The model under review builds one solid part; all positions refer to its coordinate system, in mm. A direction names the side the tool comes from. Coordinates: 2 decimals unless noted, no trailing zeros. Write each loop counter-clockwise with the first axis right and the second up, starting at its lowest first coordinate (ties: lowest second). Pieces come first, ordered by that corner, then holes. Notation, with made-up numbers: (-36.5, -2.75) - (-25.5, -2.75) arc R31 ccw to (-25.5, 34.25) - close; hole circle Ø9 at (-10, 41). An arc over 180 degrees is marked (long way). Answer as CSV lines item,"result". Start each with the question number.
```python
from build123d import *

# Parameters (mm, degrees)
SKETCH_1_R          = 2.5
EXTRUDE_1_DEPTH     = 1.5
SKETCH_3_R          = 6
EXTRUDE_2_DEPTH     = 1.5
SKETCH_4_R          = 4.5
EXTRUDE_3_DEPTH     = 6
SKETCH_5_R          = 3.25
EXTRUDE_4_DEPTH     = 1
CHAMFER_1_SIZE      = 0.5
CUT_EXTRUDE_1_REACH = 15.115
SKETCH_6_W          = 35.44
SKETCH_6_H          = 3.5


with BuildPart() as part:
    # 草图1 → 凸台-拉伸1 (new body)
    with BuildSketch(Plane.XY):
        Circle(SKETCH_1_R)
    extrude(amount=EXTRUDE_1_DEPTH)

    # 草图3 → 凸台-拉伸2 (add)
    with BuildSketch(Plane.XY.offset(1.5)):
        Circle(SKETCH_3_R)
    extrude(amount=EXTRUDE_2_DEPTH)

    # 草图4 → 凸台-拉伸3 (add)
    with BuildSketch(Plane.XY.offset(3)):
        Circle(SKETCH_4_R)
    extrude(amount=EXTRUDE_3_DEPTH)

    # 草图5 → 凸台-拉伸4 (add)
    with BuildSketch(Plane.XY.offset(9)):
        Circle(SKETCH_5_R)
    extrude(amount=EXTRUDE_4_DEPTH)

    # 倒角1
    chamfer_1_edges = [part.edges().sort_by_distance(p)[0] for p in [
        (-3.25, 0, 10),
        (-2.5, 0, 0),
    ]]
    chamfer(chamfer_1_edges, length=CHAMFER_1_SIZE)

    # 切除-拉伸1: up to this face of the body (flat: up to its plane)
    cut_extrude_1_end = Plane(part.part.faces().sort_by_distance((-5.830294373, 0, 3))[0])
    # 草图6 → 切除-拉伸1 (cut, up to the picked face)
    with BuildSketch(Plane.XY.offset(10), mode=Mode.PRIVATE) as cut_extrude_1_sk1:
        Rectangle(SKETCH_6_W, SKETCH_6_H)
    cut_extrude_1_tool1 = split(extrude(cut_extrude_1_sk1.sketch, amount=-CUT_EXTRUDE_1_REACH, mode=Mode.PRIVATE), bisect_by=cut_extrude_1_end, keep=Keep.BOTH, mode=Mode.PRIVATE)
    add(cut_extrude_1_tool1.solids().sort_by(Axis((0, 0, 10), (0, 0, -1)))[0], mode=Mode.SUBTRACT)


solid = part.part
```
(1) The part is to be moulded in two halves that separate along Z. For faces 6 (the cylindrical face through (0.1, 4.5, 6)), 7 (the conical face through (-0.04, -2.89, 9.86)), 8 (the flat face through (0, 0, 0)), say which applies: released by +Z, released by -Z, zero draft, split by the parting line, or undercut.
(2) For faces 1 (the flat face through (0, -1.75, 7)), 2 (the flat face through (-0.1, -3.4, 9)), 3 (the flat face through (-0.1, 3.4, 9)), 4 (the flat face through (0, -2, 10)), 5 (the cylindrical face through (-0.54, -2.44, 0.99)), list the 3-axis set-ups (+Z, -Z, +X, -X, +Y, -Y) from which the entire face can be reached by the end or side of a thin tool; tool diameter is ignored.
(3) For pin 1 (2 mm diameter, centred on x = -0.5, z = 7, fed in from -Y); pin 2 (1.4 mm diameter, centred on x = 0.5, y = 3.5, fed in from +Z); pin 3 (1 mm diameter, centred on x = 4, y = -2, fed in from +Z), all flat-tipped, find the tip position at first contact; note any pin that passes through.
(4) Add section C-C on x = 0. Give the boundary of the cut face in (y, z).
(5) Add section D-D on z = 1.25. Give the boundary of the cut face in (x, y).
(6) Add section B-B on y = 0. Give the boundary of the cut face in (x, z), then the cut area to 4 significant figures.
(7) Wall thickness on line 1 (Y direction, x = 0, z = 7.25); line 2 (Z direction, x = 0.25, y = 1.5); line 3 (Z direction, x = -2.5, y = 3.5): over which ranges is each line inside the solid? List them lowest first.
(8) Add section A-A on z = 7.5. Give the boundary of the cut face in (x, y), then the cut area to 3 significant figures.
Reported:
1,face 6,"zero draft"
1,face 7,"released by +Z"
1,face 8,"released by -Z"
2,face 1,"+Z, +X, -X"
2,face 2,"+Z, -Y"
2,face 3,"+Z, +Y"
2,face 4,"+Z, +X, -X, +Y, -Y"
2,face 5,"-Z"
3,pin 1,"y = -4.5"
3,pin 2,"z = 9.91"
3,pin 3,"z = 9"
4,outline,"(-6, 1.5) - (-2.5, 1.5) - (-2.5, 0.5) - (-2, 0) - (2, 0) - (2.5, 0.5) - (2.5, 1.5) - (6, 1.5) - (6, 3) - (4.5, 3) - (4.5, 9) - (3.25, 9) - (3.25, 9.5) - (2.75, 10) - (1.75, 10) - (1.75, 3) - (-1.75, 3) - (-1.75, 10) - (-2.75, 10) - (-3.25, 9.5) - (-3.25, 9) - (-4.5, 9) - (-4.5, 3) - (-6, 3) - close"
5,outline,"circle Ø5 at (0, 0)"
6,outline,"(-6, 1.5) - (-2.5, 1.5) - (-2.5, 0.5) - (-2, 0) - (2, 0) - (2.5, 0.5) - (2.5, 1.5) - (6, 1.5) - (6, 3) - (-6, 3) - close"
6,area,"25.25 mm²"
7,line 1,"-4.5 to -1.75, 1.75 to 4.5"
7,line 2,"0 to 3"
7,line 3,"1.5 to 9"
8,outline,"(-4.15, -1.75) arc R4.5 ccw to (4.15, -1.75) - close; (-4.15, 1.75) - (4.15, 1.75) arc R4.5 ccw to start"
8,area,"32.9 mm²"
